For this review, take the finished solid that the model builds, in its own axes (mm). A direction names the side the tool comes from. Round coordinates to 2 decimals unless told otherwise and drop trailing zeros. Order: outer loops, then holes, each group sorted by start corner. A loop starts at its lowest first (then second) coordinate and runs counter-clockwise, first axis right, second up. Notation, with made-up numbers: (61.5, -39) - (82.5, -39) arc R18 ccw to (82.5, -6) - close; hole circle Ø8 at (-34, 88). An arc over 180 degrees is marked (long way). One line per item, written item: value.
```python
from build123d import *

# Parameters (mm, degrees)
SKETCH2_W           = 57.15
SKETCH2_H           = 49.784
BOSS_EXTRUDE1_DEPTH = 14.224
SKETCH3_W           = 44.196
SKETCH3_H           = 39.37
CUT_EXTRUDE1_DEPTH  = 8.255
SKETCH4_W           = 35.56
SKETCH4_H           = 4.191
SKETCH4_W_2         = 15.621
SKETCH4_H_2         = 6.858
CUT_EXTRUDE2_DEPTH  = 8.255
SKETCH5_W           = 7.62
SKETCH5_H           = 8.89
SKETCH5_H_2         = 7.62
BOSS_EXTRUDE2_DEPTH = 6.604
SKETCH6_W           = 2.54
SKETCH6_H           = 5.08
SKETCH6_W_2         = 5.08
SKETCH6_H_2         = 2.54
CUT_EXTRUDE3_DEPTH  = 6.604
FILLET1_R           = 5.08
FILLET2_R           = 2.54
SKETCH7_W           = 127
SKETCH7_H           = 14.224
SKETCH7_R           = 2.38125
BOSS_EXTRUDE3_DEPTH = 5.207
BOSS_EXTRUDE4_DEPTH = 127
SKETCH11_W          = 34.925
SKETCH11_H          = 11.176
BOSS_EXTRUDE5_DEPTH = 5.207
SKETCH9_R           = 2.413
CUT_EXTRUDE4_DEPTH  = 25.4
FILLET3_R           = 5.08
FILLET4_R           = 5.08
BOSS_EXTRUDE6_DEPTH = 6.35
BOSS_EXTRUDE7_DEPTH = 6.35
BOSS_EXTRUDE8_DEPTH = 127
BOSS_EXTRUDE9_DEPTH = 127
CUT_EXTRUDE6_START  = -2.199704526
SKETCH16_R          = 2.413
CUT_EXTRUDE6_DEPTH  = 2.199704526
CUT_EXTRUDE9_START  = -17.813215
SKETCH17_R          = 5.08
CUT_EXTRUDE9_DEPTH  = 7.653215
FILLET5_R           = 3.81


with BuildPart() as part:
    # Sketch2 → Boss-Extrude1 (new body)
    with BuildSketch(Plane(origin=(0, 0, 0), x_dir=(1, 0, 0), z_dir=(0, 1, 0))):
        with Locations((28.575, 24.892)):
            Rectangle(SKETCH2_W, SKETCH2_H)
    extrude(amount=BOSS_EXTRUDE1_DEPTH)

    # Sketch3 → Cut-Extrude1 (cut)
    with BuildSketch(Plane(origin=(0, 14.224, 0), x_dir=(1, 0, 0), z_dir=(0, 1, 0))):
        with Locations((28.575, 24.892)):
            Rectangle(SKETCH3_W, SKETCH3_H)
    extrude(amount=-CUT_EXTRUDE1_DEPTH, mode=Mode.SUBTRACT)

    # Sketch4 → Cut-Extrude2 (cut)
    with BuildSketch(Plane(origin=(0, 5.969, 0), x_dir=(1, 0, 0), z_dir=(0, 1, 0))):
        with Locations((28.575, 12.5095)):
            Rectangle(SKETCH4_W, SKETCH4_H)
        with Locations((28.575, 24.638)):
            Rectangle(SKETCH4_W_2, SKETCH4_H_2)
    extrude(amount=-CUT_EXTRUDE2_DEPTH, mode=Mode.SUBTRACT)

    # Sketch5 → Boss-Extrude2 (add)
    with BuildSketch(Plane(origin=(0, 14.224, 0), x_dir=(1, 0, 0), z_dir=(0, 1, 0))):
        with Locations((-3.81, 24.765)):
            Rectangle(SKETCH5_W, SKETCH5_H)
        Polygon((12.7, 49.784), (36.83, 49.784), (44.45, 49.784), (44.45, 57.404), (36.83, 57.404), (12.7, 57.404), align=None)
        with Locations((60.96, 24.765)):
            Rectangle(SKETCH5_W, SKETCH5_H_2)
    extrude(amount=-BOSS_EXTRUDE2_DEPTH)

    # Sketch6 → Cut-Extrude3 (cut)
    with BuildSketch(Plane(origin=(0, 14.224, 0), x_dir=(1, 0, 0), z_dir=(0, 1, 0))):
        with Locations((-3.81, 24.765)):
            Rectangle(SKETCH6_W, SKETCH6_H)
        with Locations((60.96, 24.765)):
            Rectangle(SKETCH6_W, SKETCH6_H)
        with Locations((16.51, 53.594)):
            Rectangle(SKETCH6_W_2, SKETCH6_H_2)
        with Locations((40.64, 53.594)):
            Rectangle(SKETCH6_W_2, SKETCH6_H_2)
    extrude(amount=-CUT_EXTRUDE3_DEPTH, mode=Mode.SUBTRACT)

    # Fillet1
    fillet1_edges = [part.edges().sort_by_distance(p)[0] for p in [
        (0, 7.112, -49.784),
        (57.15, 7.112, -49.784),
        (57.15, 7.112, 0),
        (0, 7.112, 0),
    ]]
    fillet(fillet1_edges, radius=FILLET1_R)

    # Fillet2
    fillet2_edges = [part.edges().sort_by_distance(p)[0] for p in [
        (-7.62, 10.922, -20.32),
        (-7.62, 10.922, -29.21),
        (12.7, 10.922, -57.404),
        (44.45, 10.922, -57.404),
        (64.77, 10.922, -28.575),
        (64.77, 10.922, -20.955),
    ]]
    fillet(fillet2_edges, radius=FILLET2_R)

    # Sketch7 → Boss-Extrude3 (add)
    with BuildSketch(Plane.XY):
        with Locations((28.575, 7.112)):
            Rectangle(SKETCH7_W, SKETCH7_H)
        with Locations((-30.861, 7.112)):
            Circle(SKETCH7_R, mode=Mode.SUBTRACT)
        with Locations((88.011, 7.112)):
            Circle(SKETCH7_R, mode=Mode.SUBTRACT)
    extrude(amount=-BOSS_EXTRUDE3_DEPTH)

    # Sketch8 → Boss-Extrude4 (add)
    with BuildSketch(Plane.ZY.offset(34.925)):
        Polygon((0, 25.4), (14.664696837, 25.4), (0, 0), (-5.207, 0), (-5.207, 14.224), (0, 14.224), align=None)
    extrude(amount=-BOSS_EXTRUDE4_DEPTH)

    # Sketch11 → Boss-Extrude5 (add)
    with BuildSketch(Plane(origin=(0, 0, 0), x_dir=(-1, 0, 0), z_dir=(0, 0, -1))):
        with Locations((17.4625, 19.812)):
            Rectangle(SKETCH11_W, SKETCH11_H)
        with Locations((-74.6125, 19.812)):
            Rectangle(SKETCH11_W, SKETCH11_H)
    extrude(amount=BOSS_EXTRUDE5_DEPTH)

    # Sketch9 → Cut-Extrude4 (cut, symmetric)
    with BuildSketch(Plane(origin=(0, 0, 0), x_dir=(1, 0, 0), z_dir=(0, -0.5000000000000043, 0.8660254037844363))):
        with Locations(Location((-22.225, 11.549393675, 0), (0, 0, 270))):
            Circle(SKETCH9_R)
        with Locations(Location((79.375, 11.549393675, 0), (0, 0, 270))):
            Circle(SKETCH9_R)
    extrude(amount=CUT_EXTRUDE4_DEPTH, both=True, mode=Mode.SUBTRACT)

    # Fillet3
    fillet3_edges = [part.edges().sort_by_distance(p)[0] for p in [
        (44.45, 10.922, -49.784),
        (12.7, 10.922, -49.784),
    ]]
    fillet(fillet3_edges, radius=FILLET3_R - 0.0001)  # a hair under: the kernel refuses the full size

    # Fillet4
    fillet4_edges = [part.edges().sort_by_distance(p)[0] for p in [
        (57.15, 10.922, -20.955),
        (57.15, 10.922, -28.575),
        (0, 10.922, -29.21),
        (0, 10.922, -20.32),
    ]]
    fillet(fillet4_edges, radius=FILLET4_R - 0.0001)  # a hair under: the kernel refuses the full size

    # Sketch12 → Boss-Extrude6 (add)
    with BuildSketch(Plane.ZY):
        Polygon((-5.207, 25.4), (-15.24, 0), (-5.207, 0), align=None)
    extrude(amount=BOSS_EXTRUDE6_DEPTH)

    # Sketch13 → Boss-Extrude7 (add)
    with BuildSketch(Plane(origin=(57.15, 0, 0), x_dir=(0, 0, -1), z_dir=(1, 0, 0))):
        Polygon((5.207, 25.4), (15.875, 0), (5.207, 0), align=None)
    extrude(amount=BOSS_EXTRUDE7_DEPTH)

    # Sketch14 → Boss-Extrude8 (add)
    with BuildSketch(Plane.ZY.offset(34.925)):
        Polygon((-5.207, 0), (-5.207, -9.018788555), (0, 0), align=None)
    extrude(amount=-BOSS_EXTRUDE8_DEPTH)

    # Sketch15 → Boss-Extrude9 (add)
    with BuildSketch(Plane(origin=(92.075, 0, 0), x_dir=(0, 0, -1), z_dir=(1, 0, 0))):
        Polygon((5.207, -9.018788555), (2.667, -9.018788555), (-17.204696837, 25.4), (-14.664696837, 25.4), align=None)
    extrude(amount=-BOSS_EXTRUDE9_DEPTH)

    # Sketch16 → Cut-Extrude6 (cut)
    with BuildSketch(Plane(origin=(0, 0, 0), x_dir=(-1, 0, 0), z_dir=(0, 0.5000000000000031, -0.8660254037844369)).offset(CUT_EXTRUDE6_START)):
        with Locations(Location((-79.375, 11.549393675, 0), (0, 0, 270))):
            Circle(SKETCH16_R)
        with Locations(Location((22.225, 11.549393675, 0), (0, 0, 270))):
            Circle(SKETCH16_R)
    extrude(amount=CUT_EXTRUDE6_DEPTH, mode=Mode.SUBTRACT)

    # Sketch17 → Cut-Extrude9 (cut)
    with BuildSketch(Plane(origin=(0, -1.099852263, 1.905), x_dir=(1, 0, 0), z_dir=(0, -0.500000000000003, 0.8660254037844369)).offset(CUT_EXTRUDE9_START)):
        with Locations(Location((79.375, 11.549393675, 0), (0, 0, 90))):
            Circle(SKETCH17_R)
        with Locations(Location((-22.225, 11.549393675, 0), (0, 0, 90))):
            Circle(SKETCH17_R)
    extrude(amount=CUT_EXTRUDE9_DEPTH, mode=Mode.SUBTRACT)

    # Fillet5
    fillet5_edges = [part.edges().sort_by_distance(p)[0] for p in [
        (92.075, 25.4, 5.998848419),
        (92.075, 8.190605722, -5.207),
        (-34.925, 25.4, 5.998848419),
        (-34.925, 8.190605722, -5.207),
    ]]
    fillet(fillet5_edges, radius=FILLET5_R)


solid = part.part
```
Item 1: Machinability: for faces 4 (the flat face through (50.673, 10, -25)), 5 (the flat face through (43.18, 11, -54)), 6 (the cylindrical face through (-1.528, 10.876, -18.871)), 7 (the cylindrical face through (64.006, 10.876, -21.679)), 8 (the flat face through (0, 20, -4)), which of the approach directions +Z, -Z, +X, -X, +Y, -Y give a long, thin tool a straight path to every point of the face, cutting with its end or side? Answer none if there is none.
Returned:
face 4: +Y
face 5: +Y, -Y
face 6: -X, +Y, -Y
face 7: +X, +Y, -Y
face 8: -Z, +Y
Item 2: Take a section at D-D (z = -31.5). Write out the cut boundary in (x, y).
Returned:
outline: (-0.83, 7.62) - (0, 7.62) - (0, 0) - (57.15, 0) - (57.15, 7.62) - (57.63, 7.62) - (57.63, 14.22) - (50.67, 14.22) - (50.67, 5.97) - (6.48, 5.97) - (6.48, 14.22) - (-0.83, 14.22) - close
Item 3: Wall thickness on line 1 (Z direction, x = 22, y = 5) (3 decimals); line 2 (X direction, y = 6.5, z = -31); line 3 (Z direction, x = 39.5, y = 12.5): over which ranges is each line inside the solid? List them lowest first.
Returned:
line 1: -49.784 to -28.067, -21.209 to -14.605, -10.414 to 5.427
line 2: 0 to 6.48, 50.67 to 57.15
line 3: -57.4 to -54.86, -52.32 to -44.58, -5.21 to 9.76
Item 4: The part is to be moulded in two halves that separate along Z. For faces 1 (the flat face through (64.77, 11, -25)), 2 (the flat face through (-2.54, 11, -25)), 3 (the flat face through (28, 20, 0)), say which applies: +Z half, -Z half, draft (parallel to the pull), parting line (faces both ways), or undercut.
Returned:
face 1: draft
face 2: undercut
face 3: -Z half
Item 5: Take a section at B-B (z = -13). Write out the cut boundary in (x, y) (3 decimals), plus the area to 3 significant figures.
Returned:
outline: (-6.35, 0) - (10.795, 0) - (10.795, 5.969) - (6.477, 5.969) - (6.477, 14.224) - (0, 14.224) - (0, 5.671) - (-6.35, 5.671) - close; (46.355, 0) - (63.5, 0) - (63.5, 6.845) - (57.15, 6.845) - (57.15, 14.224) - (50.673, 14.224) - (50.673, 5.969) - (46.355, 5.969) - close
area: 315 mm^2
Item 6: For P1, Ø9, axis at x = 36, y = 21.5, coming from the -Z side; P2, Ø1.8, axis at y = 2.5, z = -26, coming from the -X side; P3, Ø2.5, axis at y = 10.5, z = -33, coming from the +X side, all flat-tipped, find the tip position at first contact; note any pin that passes through.
Returned:
P1: z = 0
P2: x = 0
P3: x = 57.52
Item 7: Take a section at A-A (x = 29.5). Write out the cut boundary in (y, z) (3 decimals), plus the area to 3 significant figures.
Returned:
outline: (-9.019, -5.207) - (0, -5.207) - (0, -10.414) - (5.969, -10.414) - (5.969, -5.207) - (14.224, -5.207) - (14.224, 0) - (25.4, 0) - (25.4, 17.205) - (-9.019, -2.667) - close; (0, -49.784) - (7.62, -49.784) - (7.62, -57.404) - (14.224, -57.404) - (14.224, -44.577) - (5.969, -44.577) - (5.969, -28.067) - (0, -28.067) - close; (0, -21.209) - (5.969, -21.209) - (5.969, -14.605) - (0, -14.605) - close
area: 665 mm^2
Item 8: Take a section at C-C (y = -4.5). Write out the cut boundary in (x, z) (3 decimals).
Returned:
outline: (-34.925, -1.397) arc R3.81 ccw to (-31.115, -5.207) - (88.265, -5.207) arc R3.81 ccw to (92.075, -1.397) - (92.075, -0.058) - (-34.925, -0.058) - close
